```python
from build123d import *
from build123d.topology import SkipClean

# Parameters (mm, degrees)
SKETCH1_R           = 1.75
BOSS_EXTRUDE1_DEPTH = 10
SKETCH2_W           = 15
SKETCH2_H           = 12.7
CUT_EXTRUDE1_DEPTH  = 4.5
FILLET1_R           = 0.5
BOSS_EXTRUDE2_START = 5
SKETCH3_R           = 3.5
SKETCH3_R_2         = 1.75
BOSS_EXTRUDE2_DEPTH = 5
SKETCH4_R           = 1.85
CUT_EXTRUDE2_DEPTH  = 33.277275288
SKETCH5_R           = 1.95
CUT_EXTRUDE3_DEPTH  = 4


with BuildPart() as part:
    # Sketch1 → Boss-Extrude1 (new body)
    with BuildSketch(Plane(origin=(0, 0, 0), x_dir=(1, 0, 0), z_dir=(0, 1, 0))):
        with BuildLine():
            Line((0, 0), (12, 0))
            ThreePointArc((12, 0), (13.5, 1.5), (15, 0))
            Line((15, 0), (15, -1.15))
            Line((15, -1.15), (25, -1.15))
            Line((25, -1.15), (25, 13.85))
            Line((25, 13.85), (15, 13.85))
            Line((15, 13.85), (15, 12.7))
            ThreePointArc((15, 12.7), (13.5, 11.2), (12, 12.7))
            Line((12, 12.7), (0, 12.7))
            Line((0, 12.7), (0, 0))
        make_face()
        with Locations(Location((5, 6.35, 0), (0, 0, 270))):
            Circle(SKETCH1_R, mode=Mode.SUBTRACT)
        with Locations(Location((20, 6.35, 0), (0, 0, 270))):
            Circle(SKETCH1_R, mode=Mode.SUBTRACT)
    extrude(amount=BOSS_EXTRUDE1_DEPTH)

    # Sketch2 → Cut-Extrude1 (cut)
    with BuildSketch(Plane(origin=(0, 10, 0), x_dir=(1, 0, 0), z_dir=(0, 1, 0))):
        with Locations((7.5, 6.35)):
            Rectangle(SKETCH2_W, SKETCH2_H)
    extrude(amount=-CUT_EXTRUDE1_DEPTH, mode=Mode.SUBTRACT)

    # Fillet1
    fillet1_edges = [part.edges().sort_by_distance(p)[0] for p in [
        (15, 5, -13.85),
        (25, 5, -13.85),
        (25, 5, 1.15),
        (12, 2.75, -12.7),
        (12, 2.75, 0),
    ]]
    fillet(fillet1_edges, radius=FILLET1_R)

    # Sketch3 → Boss-Extrude2 (add)
    with SkipClean():  # the faces are left unmerged after this step: merging them gives an invalid solid
        with BuildSketch(Plane.XZ.offset(BOSS_EXTRUDE2_START)):
            with Locations(Location((20, -6.35, 0), (0, 0, 270))):
                Circle(SKETCH3_R)
            with Locations(Location((20, -6.35, 0), (0, 0, 270))):
                Circle(SKETCH3_R_2, mode=Mode.SUBTRACT)
        extrude(amount=-BOSS_EXTRUDE2_DEPTH)

    # Sketch4 → Cut-Extrude2 (cut, through all)
    with BuildSketch(Plane.XZ.offset(5)):
        with Locations(Location((20, -6.35, 0), (0, 0, 270))):
            Circle(SKETCH4_R)
    extrude(amount=-CUT_EXTRUDE2_DEPTH, mode=Mode.SUBTRACT)

    # Sketch5 → Cut-Extrude3 (cut)
    with BuildSketch(Plane.XZ.offset(5)):
        with Locations(Location((20, -6.35, 0), (0, 0, 270))):
            Circle(SKETCH5_R)
    extrude(amount=-CUT_EXTRUDE3_DEPTH, mode=Mode.SUBTRACT)


solid = part.part
```
CAD build for the part. Positions are in the model's coordinates, mm. A direction names the side the tool comes from. Give positions to 0.01 mm unless a question says otherwise; leave off trailing zeros. Order: outer loops, then holes, each group sorted by start corner. A loop starts at its lowest first (then second) coordinate and runs counter-clockwise, first axis right, second up.
(1) Saw through at C-C, the plane y = 8.25. Give the cut face in (x, z), then the cut area to 3 significant figures.
(2) Saw through at A-A, the plane x = 20. Give the cut face in (y, z).
(3) Tool access for faces 1 (the flat face through (20, 5, 1.15)), 2 (the flat face through (7, 5.5, -6)), 3 (the flat face through (6, 3, -12.7)), 4 (the flat face through (6, 3, 0)): list every direction of +Z, -Z, +X, -X, +Y, -Y with a clear straight run to the whole face (end or side of a thin tool).
(4) Mould opens along X. For faces 5 (the cylindrical face through (21.644, -3.028, -7.398)), 6 (the flat face through (0, 3, -6)), 7 (the flat face through (12, 0, -6)), 8 (the cylindrical face through (23.47, -2.54, -5.89)) say: released by +X, released by -X, zero draft, split by the parting line, or undercut.
(5) Drill centre lines: L1, parallel to X at y = 2.8, z = -6.35; L2, parallel to Z at x = 5, y = 3.8; L3, parallel to X at y = -3.75, z = -6.35. Where is each one in solid material? Low to high.
(6) Saw through at B-B, the plane z = -6.35. Give the cut face in (x, y), then the cut area to 3 significant figures.
(7) Saw through at D-D, the plane y = 1.75. State how many separate pieces and enclosed holes the cut face has, then the cut area to 3 significant figures.
(8) Flat gauge pins, fed straight in: pin 1 (6.5 mm diameter, centred on x = 6, z = -8.5, fed in from +Y); pin 2 (4 mm diameter, centred on x = 5.5, y = 4, fed in from -Z); pin 3 (5 mm diameter, centred on x = 5, y = -2, fed in from +Z). Where does each tip first touch, or does it go through?
Results found:
1. outline: (15, -13.35) arc R0.5 ccw to (15.5, -13.85) - (24.5, -13.85) arc R0.5 ccw to (25, -13.35) - (25, 0.65) arc R0.5 ccw to (24.5, 1.15) - (15, 1.15) - close; hole circle Ø3.7 at (20, -6.35)
1. area: 139 mm2
2. outline: (-5, -9.85) - (0, -9.85) - (0, -13.85) - (10, -13.85) - (10, -8.2) - (-1, -8.2) - (-1, -8.3) - (-5, -8.3) - close; (-5, -4.4) - (-1, -4.4) - (-1, -4.5) - (10, -4.5) - (10, 1.15) - (0, 1.15) - (0, -2.85) - (-5, -2.85) - close
3. face 1: +Z, +X, -X, +Y, -Y
3. face 2: +Z, -Z, -X, +Y
3. face 3: -Z, -X, +Y, -Y
3. face 4: +Z, -X, +Y, -Y
4. face 5: undercut
4. face 6: released by -X
4. face 7: zero draft
4. face 8: split by the parting line
5. L1: x = 0 to 3.25, 6.75 to 18.15, 21.85 to 25
5. L2: z = -12.7 to -8.1, -4.6 to 0
5. L3: x = 16.5 to 18.05, 21.95 to 23.5
6. outline: (0, 0) - (3.25, 0) - (3.25, 5.5) - (0, 5.5) - close; (6.75, 0) - (16.5, 0) - (16.5, -5) - (18.05, -5) - (18.05, -1) - (18.15, -1) - (18.15, 10) - (15, 10) - (15, 5.5) - (6.75, 5.5) - close; (21.85, -1) - (21.95, -1) - (21.95, -5) - (23.5, -5) - (23.5, 0) - (25, 0) - (25, 10) - (21.85, 10) - close
6. area: 142 mm2
7. separate pieces: 1
7. enclosed holes: 2
7. area: 313 mm2
8. pin 1: stops at y = 5.5
8. pin 2: stops at z = -12.7
8. pin 3: stops at z = 0
